Check sheet for the modelled part. Datum: model origin and axes. Units: mm. A direction names the side the tool comes from. Give positions to 0.01 mm unless a question says otherwise; leave off trailing zeros. Write each loop counter-clockwise with the first axis right and the second up, starting at its lowest first coordinate (ties: lowest second). Pieces come first, ordered by that corner, then holes. Notation, with made-up numbers: (-10, 35) -> (30, 35) arc R15 cw to (30, 45) -> close; hole circle Ø8 at (8.5, 14.25). An arc over 180 degrees is marked (long way). Use a Markdown table: item, result. Add a question column.
1. Gauge pin test, flat ends, axial feed: P1, Ø1.5, axis at x = -162, y = 72.5, coming from the +Z side; P2, Ø1.2, axis at x = 302.5, y = -10, coming from the +Z side; P3, Ø19, axis at x = 265, y = -447, coming from the -Z side. Record the tip position at first contact, or that the pin passes through.
2. Cross-section at A-A (z = 26). Enter the section's corners in (x, y), then the cut area to 4 significant figures.
3. Set-up check for faces 5 (the flat face through (-270, -412.5, 51)), 6 (the flat face through (-4, -479, 25)), 7 (the flat face through (-304, -7, 25)), 8 (the flat face through (269, -410, 53)), 9 (the flat face through (235, 444, 53)): record each of +Z, -Z, +X, -X, +Y, -Y from which the full face is reachable in a straight line by a thin tool's end or side.
4. Cross-section at C-C (x = 50.5). Enter the section's corners in (y, z), then the cut area to 3 significant figures.
5. Cross-section at B-B (y = 7.5). Enter the section's corners in (x, z).
6. Scan lines: probe 1 along Y at (x, z) = (198, 35); probe 2 along X at (y, z) = (438.5, 46); probe 3 along Y at (x, z) = (-277, 50.5). Record each from-to range of solid material in increasing order. Write a range as [from, to].
7. Release check for a two-part mould opening along Z. For faces 1 (the flat face through (-301.5, -7, 25)), 2 (the flat face through (-4, 7, 0)), 3 (the flat face through (-235, 445, 53)), 4 (the flat face through (-270, -444, 65)) record: released by +Z, released by -Z, zero draft, split by the parting line, or undercut.
from build123d import *

# Parameters (mm, degrees)
F0_W     = 608
F0_H     = 958
F1_DEPTH = 65
F3_DEPTH = 25
F4_T     = -2.5


# Not quite as in the source:
# - a shell that OpenCascade refuses in one call is made with other operations: the cavity is built on its own and cut out


with BuildPart() as f1:
    # F0 (on Top) → F1 (new body)
    with BuildSketch(Plane.XY):
        Rectangle(F0_W, F0_H)
    extrude(amount=F1_DEPTH)

    # F2 (on face) → F3 (cut)
    with BuildSketch(Plane.XY.offset(65)):
        Polygon((235, 533.0333780003), (-235, 533.0333780003), (-235, 410), (-362.3474363838, 410), (-362.3474363838, -410), (-235, -410), (-235, -557.4594508362), (235, -557.4594508362), (235, -410), (358.7432372559, -410), (358.7432372559, 410), (235, 410), align=None)
    extrude(amount=-F3_DEPTH, mode=Mode.SUBTRACT)

    # F4: a shell. OpenCascade refuses it in one call, so the cavity is built on its own and cut out:
    # the body offset inwards by the wall thickness, plus a prism from it out through each open face.
    f4_core = offset(f1.part, amount=F4_T, kind=Kind.INTERSECTION, mode=Mode.PRIVATE)
    f4_exits = [f4_core.faces().sort_by_distance(p)[0] for p in [
        (0, 0, 37.5),
    ]]
    add(f4_core, mode=Mode.SUBTRACT)
    extrude(f4_exits, amount=-F4_T, mode=Mode.SUBTRACT)


solid = f1.part
Worked answers:
| question | item | result |
|---|---|---|
| 1 | P1 | stops at z = 2.5 |
| 1 | P2 | stops at z = 40 |
| 1 | P3 | stops at z = 0 |
| 2 | outline | (-304, -479) -> (304, -479) -> (304, 479) -> (-304, 479) -> close; hole (-301.5, -476.5) -> (301.5, -476.5) -> (301.5, 476.5) -> (-301.5, 476.5) -> close |
| 2 | area | 7,805 mm² |
| 3 | face 5 | none |
| 3 | face 6 | +Z, -Z, +X, -X, -Y |
| 3 | face 7 | +Z, -Z, -X, +Y, -Y |
| 3 | face 8 | +Z, +X, -X |
| 3 | face 9 | +Z, +Y, -Y |
| 4 | outline | (-479, 0) -> (479, 0) -> (479, 40) -> (476.5, 40) -> (476.5, 2.5) -> (-476.5, 2.5) -> (-476.5, 40) -> (-479, 40) -> close |
| 4 | area | 2,580 mm² |
| 5 | outline | (-304, 0) -> (304, 0) -> (304, 40) -> (301.5, 40) -> (301.5, 2.5) -> (-301.5, 2.5) -> (-301.5, 40) -> (-304, 40) -> close |
| 6 | probe 1 | y = [-479, -476.5], [476.5, 479] |
| 6 | probe 2 | x = [-304, -301.5], [-237.5, -235], [235, 237.5], [301.5, 304] |
| 6 | probe 3 | y = [-479, -476.5], [-412.5, -410], [410, 412.5], [476.5, 479] |
| 7 | face 1 | undercut |
| 7 | face 2 | released by -Z |
| 7 | face 3 | zero draft |
| 7 | face 4 | released by +Z |
